The model under review builds one solid part; all positions refer to its coordinate system, in mm. Round coordinates to 2 decimals unless told otherwise and drop trailing zeros. Write each loop counter-clockwise with the first axis right and the second up, starting at its lowest first coordinate (ties: lowest second). Pieces come first, ordered by that corner, then holes. Notation, with made-up numbers: (8.5, -25.5) -> (63.5, -25.5) arc R32 ccw to (63.5, 0.5) -> close; hole circle Ø2 at (15.5, 70). An arc over 180 degrees is marked (long way). Return JSON: item names as keys, results as strings. Group by question number.
1. Take a section at A-A, the plane x = 209. Write out the cut boundary in (y, z), then the cut area to 3 significant figures.
2. Clearance check with a flat-ended pin moving along its axis: P1, Ø11.5, axis at x = 133, y = 0, coming from the -Z side. State where the tip first meets the part, or that it passes through.
3. For line 1 along Y through (x, z) = (76, 7.25); line 2 along Y through (x, z) = (40, 1.25); line 3 along X through (y, z) = (-13, 3.5), list the stretches that pass through material, from the lowest coordinate up. Write a range as from..to.
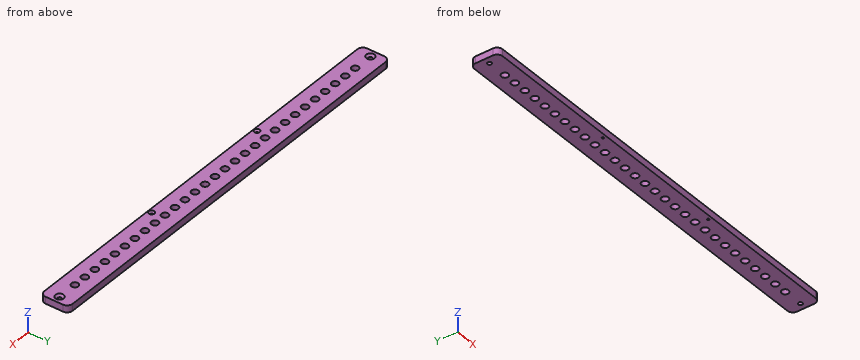
Autodesk Inventor part; units mm, degrees
ref_plane "YZ Plane" through (0, 0, 0) normal (1, 0, 0) x (0, 1, 0)
ref_plane "XZ Plane" through (0, 0, 0) normal (0, 1, 0) x (-1, 0, 0)
ref_plane "XY Plane" through (0, 0, 0) normal (0, 0, 1) x (1, 0, 0)
sketch "Sketch1" plane through (0, 0, 0) normal (0, 0, 1) x (1, 0, 0)
  line L0 (-297, 20.5) -> (297, 20.5)
  line L1 (305, 12.5) -> (305, -12.5)
  line L2 (297, -20.5) -> (-297, -20.5)
  line L3 (-305, -12.5) -> (-305, 12.5)
  arc A0 (-297, 20.5) -> (-305, 12.5) centre (-297, 12.5) ccw
  arc A1 (-305, -12.5) -> (-297, -20.5) centre (-297, -12.5) ccw
  arc A2 (305, 12.5) -> (297, 20.5) centre (297, 12.5) ccw
  arc A3 (297, -20.5) -> (305, -12.5) centre (297, -12.5) ccw
  circle A4 centre (266, 0) radius 5
  circle A5 centre (247, 0) radius 5
  circle A6 centre (228, 0) radius 5
  circle A7 centre (209, 0) radius 5
  circle A8 centre (190, 0) radius 5
  circle A9 centre (171, 0) radius 5
  circle A10 centre (152, 0) radius 5
  circle A11 centre (133, 0) radius 5
  circle A12 centre (114, 0) radius 5
  circle A13 centre (95, 0) radius 5
  circle A14 centre (76, 0) radius 5
  circle A15 centre (57, 0) radius 5
  circle A16 centre (38, 0) radius 5
  circle A17 centre (19, 0) radius 5
  circle A18 centre (0, 0) radius 5
  circle A19 centre (-19, 0) radius 5
  circle A20 centre (-38, 0) radius 5
  circle A21 centre (-57, 0) radius 5
  circle A22 centre (-76, 0) radius 5
  circle A23 centre (-95, 0) radius 5
  circle A24 centre (-114, 0) radius 5
  circle A25 centre (-133, 0) radius 5
  circle A26 centre (-152, 0) radius 5
  circle A27 centre (-171, 0) radius 5
  circle A28 centre (-190, 0) radius 5
  circle A29 centre (-209, 0) radius 5
  circle A30 centre (-228, 0) radius 5
  circle A31 centre (-247, 0) radius 5
  circle A32 centre (-266, 0) radius 5
  point P0 (305, -20.5)
  point P1 (305, 20.5)
  point P2 (-305, -20.5)
  point P3 (-305, 0)
  point P4 (0, 20.5)
  point P5 (0, 0)
  dimension "d0" = 610
  dimension "d1" = 41
  dimension "d5" = 8
  dimension "d64" = 10
  dimension "d65" = 39
  dimension "d68" = 19
extrude "Final de centella" add sketch "Sketch1" along normal blind 10
sketch "Sketch2" plane through (0, 0, 10) normal (0, 0, 1) x (1, 0, 0)
  line L0 (-295, 0) -> (295, 0) construction
  line L1 (305, -12.5) -> (305, 12.5) construction
  point P0 (0, 0)
  point P1 (0, 0)
  dimension "d10" = 590
hole "Fijación M6" at (-295, 0, 10) at (295, 0, 10) direction (0, 0, -1) diameter 6 end through all countersink diameter 12 countersink angle 90
sketch "Sketch3" plane through (0, 0, 10) normal (0, 0, 1) x (1, 0, 0)
  line L0 (132, 16) -> (266, 16) construction
  line L1 (266, 16) -> (266, -16) construction
  line L2 (305, -12.5) -> (305, 12.5) construction
  line L3 (-21, 16) -> (113, 16) construction
  line L4 (113, 16) -> (113, -16) construction
  line L5 (-174, 16) -> (-40, 16) construction
  line L6 (-40, 16) -> (-40, -16) construction
  line L7 (-325.5, 16) -> (-191.5, 16) construction
  line L8 (-191.5, 16) -> (-191.5, -16) construction
  point P0 (0, 0)
  point P1 (199, -16)
  point P2 (199, 16)
  point P3 (132, -16)
  point P4 (199, 16)
  point P5 (266, 0)
  point P6 (46, -16)
  point P7 (46, 16)
  point P8 (-21, -16)
  point P9 (46, 16)
  point P10 (113, 0)
  point P11 (-107, -16)
  point P12 (-107, 16)
  point P13 (-174, -16)
  point P14 (-107, 16)
  point P15 (-40, 0)
  point P16 (-258.5, -16)
  point P17 (-258.5, 16)
  point P18 (-325.5, -16)
  point P19 (-258.5, 16)
  point P20 (-191.5, 0)
  dimension "d22" = 32
  dimension "d23" = 134
  dimension "d24" = 39
  dimension "d26" = 134
  dimension "d27" = 19
  dimension "d29" = 134
  dimension "d30" = 19
  dimension "d32" = 134
  dimension "d33" = 17.5
hole "Fijacion M3 SiPM" [suppressed]
sketch "Sketch6" plane through (0, 0, 10) normal (0, 0, -1) x (-1, 0, 0)
  line L0 (-100, -15.5) -> (100, -15.5) construction
  line L1 (297, -20.5) -> (-297, -20.5) construction
  point P0 (0, 0)
  point P1 (0, -15.5)
  dimension "d73" = 200
  dimension "d74" = 5
hole "Ø4 M4 T madera" at (100, -15.5, 10) at (-100, -15.5, 10) direction (0, 0, -1) diameter 3 end through all countersink diameter 8 countersink angle 90
sketch "Sketch7" plane through (0, 0, 10) normal (0, 0, 1) x (1, 0, 0)
  circle A0 centre (-266, 0) radius 5
  circle A1 centre (-247, 0) radius 5
  circle A2 centre (-228, 0) radius 5
  circle A3 centre (-209, 0) radius 5
  circle A4 centre (-190, 0) radius 5
  circle A5 centre (-171, 0) radius 5
  circle A6 centre (-152, 0) radius 5
  circle A7 centre (-133, 0) radius 5
  circle A8 centre (-114, 0) radius 5
  circle A9 centre (-95, 0) radius 5
  circle A10 centre (-76, 0) radius 5
  circle A11 centre (-57, 0) radius 5
  circle A12 centre (-38, 0) radius 5
  circle A13 centre (-19, 0) radius 5
  circle A14 centre (0, 0) radius 5
  circle A15 centre (19, 0) radius 5
  circle A16 centre (38, 0) radius 5
  circle A17 centre (57, 0) radius 5
  circle A18 centre (76, 0) radius 5
  circle A19 centre (95, 0) radius 5
  circle A20 centre (114, 0) radius 5
  circle A21 centre (133, 0) radius 5
  circle A22 centre (152, 0) radius 5
  circle A23 centre (171, 0) radius 5
  circle A24 centre (190, 0) radius 5
  circle A25 centre (209, 0) radius 5
  circle A26 centre (228, 0) radius 5
  circle A27 centre (247, 0) radius 5
  circle A28 centre (266, 0) radius 5
  point P0 (0, 0)
hole "M12x1.75" at (-266, 0, 10) at (-247, 0, 10) at (-228, 0, 10) at (-209, 0, 10) at (-190, 0, 10) at (-171, 0, 10) at (-152, 0, 10) at (-133, 0, 10) at (-114, 0, 10) at (-95, 0, 10) at (-76, 0, 10) at (-57, 0, 10) at (-38, 0, 10) at (-19, 0, 10) at (0, 0, 10) at (19, 0, 10) at (38, 0, 10) at (57, 0, 10) at (76, 0, 10) at (95, 0, 10) at (114, 0, 10) at (133, 0, 10) at (152, 0, 10) at (171, 0, 10) at (190, 0, 10) at (209, 0, 10) at (228, 0, 10) at (247, 0, 10) at (266, 0, 10) direction (0, 0, -1) diameter 10.106 end through all
equation "\"d26\" = d23"
equation "\"d29\" = d23"
equation "\"d30\" = d27"
equation "\"d32\" = d23"
properties part number "Extremo centella-IN" material "PMMA Plastic"
Output:
{
 "1": {"outline": "(-20.5, 0) -> (-5.05, 0) -> (-5.05, 10) -> (-20.5, 10) -> close; (5.05, 0) -> (20.5, 0) -> (20.5, 10) -> (5.05, 10) -> close", "area": "309 mm^2"},
 "2": {"P1": "stops at z = 0"},
 "3": {"line 1": "y = -20.5..-5.05, 5.05..20.5", "line 2": "y = -20.5..-4.64, 4.64..20.5", "line 3": "x = -304.98..304.98"}
}
